from build123d import *

# Parameters (mm, degrees)
SKETCH1_W           = 21
SKETCH1_H           = 21
BOSS_EXTRUDE1_DEPTH = 4
SKETCH2_W           = 9.5
SKETCH2_H           = 9.5
BOSS_EXTRUDE2_DEPTH = 3.7
SKETCH3_W           = 14
SKETCH3_H           = 14
BOSS_EXTRUDE3_DEPTH = 3.3
FILLET1_R           = 2
FILLET2_R           = 2
FILLET3_R           = 2


with BuildPart() as part:
    # Sketch1 → Boss-Extrude1 (new body)
    with BuildSketch(Plane(origin=(0, 0, 0), x_dir=(1, 0, 0), z_dir=(0, 1, 0))):
        Rectangle(SKETCH1_W, SKETCH1_H)
    extrude(amount=BOSS_EXTRUDE1_DEPTH)

    # Sketch2 → Boss-Extrude2 (add)
    with BuildSketch(Plane.XZ):
        Rectangle(SKETCH2_W, SKETCH2_H)
    extrude(amount=BOSS_EXTRUDE2_DEPTH)

    # Sketch3 → Boss-Extrude3 (add)
    with BuildSketch(Plane(origin=(0, 4, 0), x_dir=(1, 0, 0), z_dir=(0, 1, 0))):
        Rectangle(SKETCH3_W, SKETCH3_H)
    extrude(amount=BOSS_EXTRUDE3_DEPTH)

    # Fillet1
    fillet1_edges = [part.edges().sort_by_distance(p)[0] for p in [
        (10.5, 2, 10.5),
        (-10.5, 2, 10.5),
        (-10.5, 2, -10.5),
        (10.5, 2, -10.5),
    ]]
    fillet(fillet1_edges, radius=FILLET1_R)

    # Fillet2
    fillet2_edges = [part.edges().sort_by_distance(p)[0] for p in [
        (7, 5.65, 7),
        (7, 5.65, -7),
        (-7, 5.65, -7),
        (-7, 5.65, 7),
        (7, 7.3, 0),
        (0, 7.3, -7),
        (-7, 7.3, 0),
        (0, 7.3, 7),
    ]]
    fillet(fillet2_edges, radius=FILLET2_R)

    # Fillet3
    fillet3_edges = [part.edges().sort_by_distance(p)[0] for p in [
        (4.75, -1.85, -4.75),
        (4.75, -1.85, 4.75),
        (-4.75, -1.85, 4.75),
        (-4.75, -1.85, -4.75),
        (4.75, -3.7, 0),
        (0, -3.7, 4.75),
        (-4.75, -3.7, 0),
        (0, -3.7, -4.75),
    ]]
    fillet(fillet3_edges, radius=FILLET3_R)


solid = part.part
Geometry: final body of the model. Coordinates: model frame, mm. A direction names the side the tool comes from. Round coordinates to 2 decimals unless told otherwise and drop trailing zeros. Loops run counter-clockwise (first coordinate to the right, second up) from the corner with the lowest first, then second, coordinate; pieces in that order, holes last. Notation, with made-up numbers: (40.25, 33) - (54.25, 33) arc R16 cw to (54.25, 56) - close; hole circle Ø9 at (8.25, 65). An arc over 180 degrees is marked (long way). Write each question's results on one line, items separated by ' | '. Start each with the question number.
1) Access query for faces 1 (the face through (-6.4, 4.66, 6.43)), 2 (the face through (-5, 0, 0)), 3 (the face through (-7, 5, 0)). Directions: +Z, -Z, +X, -X, +Y, -Y. A direction counts if a zero-diameter tool reaches every point of the face in a straight line with its end or side. Return the directions, or none.
2) Cut plane C-C on y = 4.75. Return loops of the section in (x, z).
3) First-contact query: P1, Ø1.4, axis at x = 0, y = -1, coming from the +Z side; P2, Ø1.5, axis at x = -3, z = -7.5, coming from the +Y side; P3, Ø0.9, axis at y = -1, z = 0.5, coming from the -X side. Flat tips, straight axial feed; report the tip coordinate or a pass-through.
4) Line query: probe 1 along Y at (x, z) = (-9.5, 7); probe 2 along Z at (x, y) = (-0.5, -1.5); probe 3 along X at (y, z) = (4.25, 0.75). Output: solid intervals per line, ascending. Write a range as [from, to].
5) Cut plane D-D on z = -5.5. Return loops of the section in (x, y), then the cut area to 3 significant figures.
6) Cut plane A-A on x = -0.5. Return loops of the section in (y, z).
7) Cut plane B-B on z = 0. Return loops of the section in (x, y).
Verdict:
1) face 1: +Z, -X, +Y | face 2: -Y | face 3: +Z, -Z, -X, +Y
2) outline: (-7, -5) arc R2 ccw to (-5, -7) - (5, -7) arc R2 ccw to (7, -5) - (7, 5) arc R2 ccw to (5, 7) - (-5, 7) arc R2 ccw to (-7, 5) - close
3) P1: stops at z = 4.75 | P2: stops at y = 6.27 | P3: stops at x = -4.75
4) probe 1: y = [0, 4] | probe 2: z = [-4.75, 4.75] | probe 3: x = [-7, 7]
5) outline: (-10.5, 0) - (10.5, 0) - (10.5, 4) - (6.94, 4) - (6.94, 5.3) arc R1.94 ccw to (5, 7.24) - (-5, 7.24) arc R1.94 ccw to (-6.94, 5.3) - (-6.94, 4) - (-10.5, 4) - close | area: 127 mm2
6) outline: (-3.7, -2.75) arc R2 ccw to (-1.7, -4.75) - (0, -4.75) - (0, -10.5) - (4, -10.5) - (4, -7) - (5.3, -7) arc R2 ccw to (7.3, -5) - (7.3, 5) arc R2 ccw to (5.3, 7) - (4, 7) - (4, 10.5) - (0, 10.5) - (0, 4.75) - (-1.7, 4.75) arc R2 ccw to (-3.7, 2.75) - close
7) outline: (-10.5, 0) - (-4.75, 0) - (-4.75, -1.7) arc R2 ccw to (-2.75, -3.7) - (2.75, -3.7) arc R2 ccw to (4.75, -1.7) - (4.75, 0) - (10.5, 0) - (10.5, 4) - (7, 4) - (7, 5.3) arc R2 ccw to (5, 7.3) - (-5, 7.3) arc R2 ccw to (-7, 5.3) - (-7, 4) - (-10.5, 4) - close
